from build123d import *

# Parameters (mm, degrees)
CYLINDER003_R     = 2
CYLINDER003_DEPTH = 2
BOX002_W          = 6.8
BOX002_H          = 2
BOX002_DEPTH      = 8
CYLINDER002_R     = 4
CYLINDER002_DEPTH = 2
CYLINDER001_R     = 2.3
CYLINDER001_DEPTH = 2
CYLINDER_R        = 4
CYLINDER_DEPTH    = 2
BOX_W             = 45
BOX_H             = 2
BOX_DEPTH         = 8
CYLINDER005_R     = 2
CYLINDER005_DEPTH = 2
BOX003_W          = 6.8
BOX003_H          = 2
BOX003_DEPTH      = 8
CYLINDER004_R     = 4
CYLINDER004_DEPTH = 2
BOX001_W          = 2
BOX001_H          = 11.6
BOX001_DEPTH      = 8


with BuildPart() as cylinder003:
    # Cylinder003 → Cylinder003 (new body)
    with BuildSketch(Plane(origin=(54, 6.8, 4), x_dir=(1, 0, 0), z_dir=(0, -1, 0))):
        Circle(CYLINDER003_R)
    extrude(amount=CYLINDER003_DEPTH)


with BuildPart() as cube002:
    # Box002 → Box002 (new body)
    with BuildSketch(Plane(origin=(47, 4.8, 0), x_dir=(1, 0, 0), z_dir=(0, 0, 1))):
        with Locations((3.4, 1)):
            Rectangle(BOX002_W, BOX002_H)
    extrude(amount=BOX002_DEPTH)


with BuildPart() as cut001:
    # Cylinder002 → Cylinder002 (new body)
    with BuildSketch(Plane(origin=(54, 6.8, 4), x_dir=(1, 0, 0), z_dir=(0, -1, 0))):
        Circle(CYLINDER002_R)
    extrude(amount=CYLINDER002_DEPTH)

    # Fusion001: union Cube002
    add(cube002.part)

    # Cut001: cut Cylinder003
    add(cylinder003.part, mode=Mode.SUBTRACT)


with BuildPart() as cylinder001:
    # Cylinder001 → Cylinder001 (new body)
    with BuildSketch(Plane(origin=(0, 2, 4), x_dir=(1, 0, 0), z_dir=(0, -1, 0))):
        Circle(CYLINDER001_R)
    extrude(amount=CYLINDER001_DEPTH)


with BuildPart() as cylinder:
    # Cylinder → Cylinder (new body)
    with BuildSketch(Plane(origin=(0, 0, 4), x_dir=(1, 0, 0), z_dir=(0, 1, 0))):
        Circle(CYLINDER_R)
    extrude(amount=CYLINDER_DEPTH)


with BuildPart() as cut:
    # Box → Box (new body)
    with BuildSketch(Plane.XY):
        with Locations((22.5, 1)):
            Rectangle(BOX_W, BOX_H)
    extrude(amount=BOX_DEPTH)

    # Fusion: union Cylinder
    add(cylinder.part)

    # Cut: cut Cylinder001
    add(cylinder001.part, mode=Mode.SUBTRACT)


with BuildPart() as cylinder005:
    # Cylinder005 → Cylinder005 (new body)
    with BuildSketch(Plane(origin=(54, 6.8, 4), x_dir=(1, 0, 0), z_dir=(0, -1, 0))):
        Circle(CYLINDER005_R)
    extrude(amount=CYLINDER005_DEPTH)


with BuildPart() as cube003:
    # Box003 → Box003 (new body)
    with BuildSketch(Plane(origin=(47, 4.8, 0), x_dir=(1, 0, 0), z_dir=(0, 0, 1))):
        with Locations((3.4, 1)):
            Rectangle(BOX003_W, BOX003_H)
    extrude(amount=BOX003_DEPTH)


with BuildPart() as cut002:
    # Cylinder004 → Cylinder004 (new body)
    with BuildSketch(Plane(origin=(54, 6.8, 4), x_dir=(1, 0, 0), z_dir=(0, -1, 0))):
        Circle(CYLINDER004_R)
    extrude(amount=CYLINDER004_DEPTH)

    # Fusion002: union Cube003
    add(cube003.part)

    # Cut002: cut Cylinder005
    add(cylinder005.part, mode=Mode.SUBTRACT)


with BuildPart() as cut002_1:
    # Cut002 placement: moved
    add(cut002.part.moved(Location((0, -9.6, 0))))


with BuildPart() as fusion003:
    # Box001 → Box001 (new body)
    with BuildSketch(Plane(origin=(45, -4.8, 0), x_dir=(1, 0, 0), z_dir=(0, 0, 1))):
        with Locations((1, 5.8)):
            Rectangle(BOX001_W, BOX001_H)
    extrude(amount=BOX001_DEPTH)

    # Fusion003: union Cut001, Cut, Cut002
    add(cut001.part)
    add(cut.part)
    add(cut002_1.part)


solid = fusion003.part
Check sheet for the modelled part. Datum: model origin and axes. Units: mm. A direction names the side the tool comes from. Round coordinates to 2 decimals unless told otherwise and drop trailing zeros. Loops run counter-clockwise (first coordinate to the right, second up) from the corner with the lowest first, then second, coordinate; pieces in that order, holes last. Notation, with made-up numbers: M 1.25,29.25 L 47.25,29.25 A23 ccw 47.25,63.25 Z; hole C 82.5,10.25 d9. An arc over 180 degrees is marked long. One line per question, with ' | ' between items. Start each with the question number.
Item 1: Section check B-B (z = 4). Record the boundary of the cut face in (x, y).
Item 2: Section check C-C (y = -1.75). Record the boundary of the cut face in (x, z), and give its area (3 significant figures).
Item 3: Scan lines: probe 1 along Y at (x, z) = (52, 3.25); probe 2 along Z at (x, y) = (54, 6); probe 3 along Y at (x, z) = (38.5, 1). Record each from-to range of solid material in increasing order.
Item 4: Gauge pin test, flat ends, axial feed: pin 1 Ø1.5 at (y, z) = (5.5, 3.5) entering from -X; pin 2 Ø2.5 at (x, z) = (52.5, 5) entering from -Y; pin 3 Ø1 at (y, z) = (2, 3.5) entering from +X; pin 4 Ø4 at (x, z) = (32, 3) entering from -Y. Record the tip position at first contact, or that the pin passes through.
Item 5: Set-up check for faces 1 (the face through (45, 4, 4)), 2 (the face through (51, -2.8, 4)), 3 (the face through (20, 0, 4)), 4 (the face through (-4, 1, 4)): record each of +Z, -Z, +X, -X, +Y, -Y from which the full face is reachable in a straight line by a thin tool's end or side.
Item 6: Release check for a two-part mould opening along Y. For faces 5 (the face through (50, -4.8, 4)), 6 (the face through (55.847, 5.814, 3.234)), 7 (the face through (51, 4.8, 4)) record: released by +Y, released by -Y, zero draft, split by the parting line, or undercut.
Item 7: Section check A-A (x = 49.5). Record the boundary of the cut face in (y, z), and give its area (3 significant figures).
Item 8: Section check D-D (x = 37). Record the boundary of the cut face in (y, z).
Worked out:
1) outline: M -4,0 L -2.3,0 L -2.3,2 L -4,2 Z; M 2.3,0 L 45,0 L 45,-4.8 L 52,-4.8 L 52,-2.8 L 47,-2.8 L 47,4.8 L 52,4.8 L 52,6.8 L 45,6.8 L 45,2 L 2.3,2 Z; M 56,-4.8 L 58,-4.8 L 58,-2.8 L 56,-2.8 Z; M 56,4.8 L 58,4.8 L 58,6.8 L 56,6.8 Z
2) outline: M 45,0 L 47,0 L 47,8 L 45,8 Z | area: 16.0 mm^2
3) probe 1: -4.8 to -2.8, 4.8 to 6.8 | probe 2: 0 to 2, 6 to 8 | probe 3: 0 to 2
4) pin 1: x = 45 | pin 2: y = -4.8 | pin 3: x = 47 | pin 4: y = 0
5) face 1: +Z, -Z, -X, +Y | face 2: +Z, -Z, +X | face 3: +Z, -Z, -X, -Y | face 4: -X, +Y, -Y
6) face 5: released by -Y | face 6: zero draft | face 7: undercut
7) outline: M -4.8,0 L -2.8,0 L -2.8,8 L -4.8,8 Z; M 4.8,0 L 6.8,0 L 6.8,8 L 4.8,8 Z | area: 32.0 mm^2
8) outline: M 0,0 L 2,0 L 2,8 L 0,8 Z
